Here's how the part is built. I have some questions about the finished solid (model axes, mm). Round coordinates to 2 decimals unless told otherwise and drop trailing zeros. Use a Markdown table: item, result. Add a question column.
(1) If I drill on probe 1 along Y at (x, z) = (0, -0.45); probe 2 along Y at (x, z) = (-2, -1.25); probe 3 along X at (y, z) = (98.5, 0.15), over which ranges is the centre line in solid material (lowest first)?
(2) I want a section at A-A, the plane z = -0.4. Give the number of separate pieces and of enclosed holes in the cut face, then the cut area to 3 significant figures.
(3) I'm going to push flat-ended pins straight in: P1, Ø2, axis at y = 9, z = 0.5, coming from the +X side; P2, Ø1, axis at y = 30.5, z = 0, coming from the +X side. Where does each tip first touch, or does it pass through?
from build123d import *

# Parameters (mm, degrees)
BOSS_EXTRUDE1_START       = -2
BOSS_EXTRUDE1_OUTLINE_R   = 4
BOSS_EXTRUDE1_OUTLINE_R_2 = 5
BOSS_EXTRUDE1_OUTLINE_R_3 = 1
BOSS_EXTRUDE1_DEPTH       = 4
FILLET1_R                 = 0.8


# Read off the part's stored shape, not the designer's step: Boss-Extrude1
with BuildPart() as part:
    # Boss-Extrude1 outline → Boss-Extrude1 (new body)
    with BuildSketch(Plane.XY.offset(BOSS_EXTRUDE1_START)):
        with BuildLine():
            ThreePointArc((-4.09240869, 3.386100226), (-1.799457661, -4.997542972), (5.311636624, 0))
            add(Edge.make_bspline(
                [(5.311636624, 0), (17.769363539, 34.421881869), (25.192042954, 73.13636609), (16.37011227, 109.364122199)],
                knots=[0, 0, 0, 0, 0.956773453, 0.956773453, 0.956773453, 0.956773453], degree=3))
            ThreePointArc((16.37011227, 109.364122199), (6.842083232, 120.574345754), (5.817157068, 105.897766593))
            add(Edge.make_bspline(
                [(-4.09240869, 3.386100226), (6.994812741, 21.577875377), (13.208144478, 57.701592599), (9.143863643, 92.456079954), (5.817157068, 105.897766593)],
                knots=[0, 0, 0, 0, 0.587614162, 0.97029995, 0.97029995, 0.97029995, 0.97029995], degree=3))
        make_face()
        Circle(BOSS_EXTRUDE1_OUTLINE_R, mode=Mode.SUBTRACT)
        with Locations((9.321130613, 113.027146637)):
            Circle(BOSS_EXTRUDE1_OUTLINE_R_2, mode=Mode.SUBTRACT)
        with Locations((11.949864601, 104.478258332)):
            Circle(BOSS_EXTRUDE1_OUTLINE_R_3, mode=Mode.SUBTRACT)
    extrude(amount=BOSS_EXTRUDE1_DEPTH)

    # Fillet1
    fillet1_edges = [part.edges().sort_by_distance(p)[0] for p in [
        (4.321130613, 113.027146637, -2),
        (-4, 0, -2),
        (-4, 0, 2),
        (4.321130613, 113.027146637, 2),
    ]]
    fillet(fillet1_edges, radius=FILLET1_R)


solid = part.part
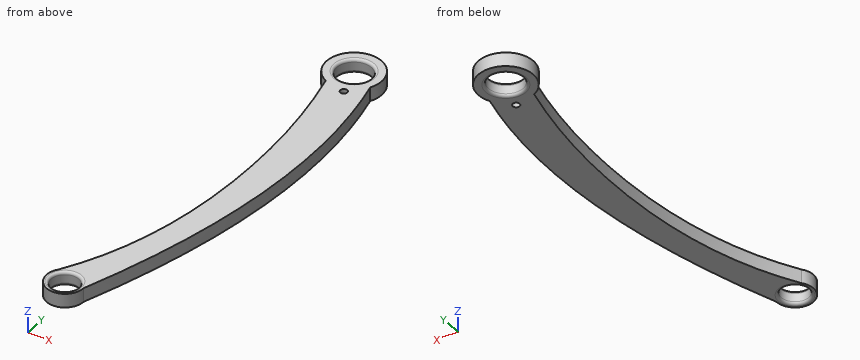
Taken from the geometry:
| question | item | result |
|---|---|---|
| 1 | probe 1 | y = -5.31 to -4, 4 to 10.93 |
| 1 | probe 2 | y = -4.92 to -3.47, 3.47 to 7.02 |
| 1 | probe 3 | x = 7.47 to 18.53 |
| 2 | separate pieces | 1 |
| 2 | enclosed holes | 3 |
| 2 | area | 1,090 mm2 |
| 3 | P1 | stops at x = 8.74 |
| 3 | P2 | stops at x = 14.64 |
